```python
from build123d import *

# Parameters (mm, degrees)
SKETCH_W      = 34
SKETCH_H      = 32
SKETCH_R      = 2.5
SKETCH_R_2    = 11.1
PAD_DEPTH     = 7
SKETCH001_W   = 34
SKETCH001_H   = 32
SKETCH001_R   = 2.5
SKETCH001_R_2 = 9
PAD001_DEPTH  = 2
FILLET_R      = 2


with BuildPart() as part:
    # Sketch → Pad (new body)
    with BuildSketch(Plane.XY):
        Rectangle(SKETCH_W, SKETCH_H)
        with Locations((-9.2, 10.5)):
            Circle(SKETCH_R, mode=Mode.SUBTRACT)
        with Locations((9.2, 10.5)):
            Circle(SKETCH_R, mode=Mode.SUBTRACT)
        with Locations((-9.2, -10.5)):
            Circle(SKETCH_R, mode=Mode.SUBTRACT)
        with Locations((9.2, -10.5)):
            Circle(SKETCH_R, mode=Mode.SUBTRACT)
        Circle(SKETCH_R_2, mode=Mode.SUBTRACT)
    extrude(amount=PAD_DEPTH)

    # Sketch001 → Pad001 (join)
    with BuildSketch(Plane.XY):
        Rectangle(SKETCH001_W, SKETCH001_H)
        with Locations((-9.2, 10.5)):
            Circle(SKETCH001_R, mode=Mode.SUBTRACT)
        with Locations((9.2, 10.5)):
            Circle(SKETCH001_R, mode=Mode.SUBTRACT)
        with Locations((-9.2, -10.5)):
            Circle(SKETCH001_R, mode=Mode.SUBTRACT)
        with Locations((9.2, -10.5)):
            Circle(SKETCH001_R, mode=Mode.SUBTRACT)
        Circle(SKETCH001_R_2, mode=Mode.SUBTRACT)
    extrude(amount=-PAD001_DEPTH)

    # Fillet
    fillet_edges = [part.edges().sort_by_distance(p)[0] for p in [
        (17, -16, -1),
        (17, -16, 3.5),
        (-17, -16, -1),
        (-17, -16, 3.5),
        (17, 16, 3.5),
        (17, 16, -1),
        (-17, 16, 3.5),
        (-17, 16, -1),
    ]]
    fillet(fillet_edges, radius=FILLET_R)


solid = part.part
```
Geometry: final body of the model. Coordinates: model frame, mm. A direction names the side the tool comes from. Round coordinates to 2 decimals unless told otherwise and drop trailing zeros. Order: outer loops, then holes, each group sorted by start corner. A loop starts at its lowest first (then second) coordinate and runs counter-clockwise, first axis right, second up. Notation, with made-up numbers: M 81.5,40.5 L 113.5,40.5 A33 ccw 113.5,68.5 Z; hole C 20,-20.5 d10. An arc over 180 degrees is marked long. Use one line per item in the form item = value. Start each with the question number.
Q1. Pin query (flat end, axial travel): pin 1 Ø6.5 at (x, y) = (-4.5, -4.5) entering from +Z. Return the tip coordinate at first contact, or that it passes through.
Q2. Cut plane A-A (x = 0). Return loops of the section in (y, z).
Q3. Cut plane C-C (z = 5.5). Return loops of the section in (x, y).
Q4. Cut plane D-D (y = -10.5). Return loops of the section in (x, z), and give its area (3 significant figures).
Q5. Access query for faces 4 (the face through (-17, 0, 3)), 5 (the face through (-2, 9, 0)). Directions: +Z, -Z, +X, -X, +Y, -Y. A direction counts if a zero-diameter tool reaches every point of the face in a straight line with its end or side. Return the directions, or none.
Q6. Mould query, pull axis X, two halves, no side actions, for faces 1 (the face through (16.43, -15.4, 2.56)), 2 (the face through (5.97, 9.36, 3.45)), 3 (the face through (-16.43, -15.4, 2.56)). Classes: +X half, -X half, draft (parallel to the pull), parting line (faces both ways), or undercut.
Q7. Cut plane B-B (y = 0). Return loops of the section in (x, z), and give its area (3 significant figures).
Q8. Material intervals for line 1 (Y direction, x = -9.2, z = -1.1); line 2 (Y direction, x = -6.5, z = 3); line 3 (Y direction, x = 0, z = 2), sorted ascending. Write a range as [from, to].
Geometry results:
q1.pin_1 = 0
q2.outline = M -16,-2 L -9,-2 L -9,0 L -11.1,0 L -11.1,7 L -16,7 Z; M 9,-2 L 16,-2 L 16,7 L 11.1,7 L 11.1,0 L 9,0 Z
q3.outline = M -17,-14 A2 ccw -15,-16 L 15,-16 A2 ccw 17,-14 L 17,14 A2 ccw 15,16 L -15,16 A2 ccw -17,14 Z; hole C -9.2,-10.5 d5; hole C -9.2,10.5 d5; hole C 0,0 d22.2; hole C 9.2,-10.5 d5; hole C 9.2,10.5 d5
q4.outline = M -17,-2 L -11.7,-2 L -11.7,7 L -17,7 Z; M -6.7,-2 L 6.7,-2 L 6.7,7 L 3.6,7 L 3.6,0 L -3.6,0 L -3.6,7 L -6.7,7 Z; M 11.7,-2 L 17,-2 L 17,7 L 11.7,7 Z
q4.area = 166 mm^2
q5.face_4 = +Z, -Z, -X, +Y, -Y
q5.face_5 = +Z
q6.face_1 = +X half
q6.face_2 = undercut
q6.face_3 = -X half
q7.outline = M -17,-2 L -9,-2 L -9,0 L -11.1,0 L -11.1,7 L -17,7 Z; M 9,-2 L 17,-2 L 17,7 L 11.1,7 L 11.1,0 L 9,0 Z
q7.area = 115 mm^2
q8.line_1 = [-16, -13], [-8, 8], [13, 16]
q8.line_2 = [-16, -9], [9, 16]
q8.line_3 = [-16, -11.1], [11.1, 16]
